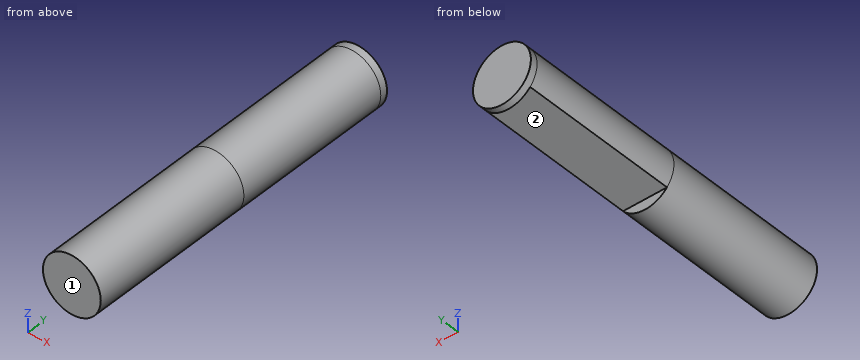
```python
from build123d import *

# Parameters (mm, degrees)
SKETCH1_R           = 8
BOSS_EXTRUDE1_DEPTH = 46
BOSS_EXTRUDE2_DEPTH = 44
SKETCH3_R           = 8
BOSS_EXTRUDE3_DEPTH = 2


with BuildPart() as part:
    # Sketch1 → Boss-Extrude1 (new body)
    with BuildSketch(Plane(origin=(0, 0, 0), x_dir=(1, 0, 0), z_dir=(0, 1, 0))):
        Circle(SKETCH1_R)
    extrude(amount=BOSS_EXTRUDE1_DEPTH)

    # Sketch2 → Boss-Extrude2 (add)
    with BuildSketch(Plane(origin=(0, 46, 0), x_dir=(1, 0, 0), z_dir=(0, 1, 0))):
        with BuildLine():
            Line((-6.079473661, 5.2), (6.079473661, 5.2))
            ThreePointArc((6.079473661, 5.2), (0, -8), (-6.079473661, 5.2))
        make_face()
    extrude(amount=BOSS_EXTRUDE2_DEPTH)

    # Sketch3 → Boss-Extrude3 (add)
    with BuildSketch(Plane(origin=(0, 90, 0), x_dir=(1, 0, 0), z_dir=(0, 1, 0))):
        Circle(SKETCH3_R)
    extrude(amount=BOSS_EXTRUDE3_DEPTH)


solid = part.part
```
Model file for the job. Use its own axes, mm. Face numbers are marked on the shaded views. A direction names the side the tool comes from. Round coordinates to 2 decimals unless told otherwise and drop trailing zeros. Write each loop counter-clockwise with the first axis right and the second up, starting at its lowest first coordinate (ties: lowest second). Pieces come first, ordered by that corner, then holes. Notation, with made-up numbers: (43.5, -31.5) - (87.5, -31.5) arc R31 ccw to (87.5, 1.5) - close; hole circle Ø7 at (-15, 31.25). An arc over 180 degrees is marked (long way). Use CSV: the item, a comma, the result in double quotes. Start each with the question number.
Item 1: Drill centre lines: L1, parallel to Y at x = -3.75, z = -6; L2, parallel to Z at x = -4, y = 18; L3, parallel to X at y = 8, z = 3.5. Where is each one in solid material? Low to high. Write a range as [from, to].
Item 2: Tool access for the marked faces 1 and 2: list every direction of +Z, -Z, +X, -X, +Y, -Y with a clear straight run to the whole face (end or side of a thin tool).
Item 3: Pin check, flat tips, straight feed: P1, Ø3, axis at x = 2, z = -7, coming from the -Y side; P2, Ø1.5, axis at y = 73.5, z = 1, coming from the -X side; P3, Ø6, axis at x = -6, y = 33.5, coming from the +Z side; P4, Ø1.5, axis at y = 59.5, z = -2.5, coming from the -X side. Stop position of each tip, or through.
Item 4: Band-saw the part on B-B (y = 8.5). Write the cut outline in (x, z).
Item 5: Band-saw the part on A-A (x = 0). Write the cut outline in (y, z).
Item 6: Band-saw the part on D-D (z = 1.75). Write the cut outline in (x, y), and give its area (3 significant figures).
Item 7: Band-saw the part on C-C (z = 6). Write the cut outline in (x, y).
Checked values:
1,L1,"y = [0, 46], [90, 92]"
1,L2,"z = [-6.93, 6.93]"
1,L3,"x = [-7.19, 7.19]"
2,face 1,"+Z, -Z, +X, -X, -Y"
2,face 2,"-Z, +X, -X"
3,P1,"stops at y = 0"
3,P2,"stops at x = -8"
3,P3,"stops at z = 7.42"
3,P4,"stops at x = -7.81"
4,outline,"circle Ø16 at (0, 0)"
5,outline,"(0, -8) - (46, -8) - (46, -5.2) - (90, -5.2) - (90, -8) - (92, -8) - (92, 8) - (0, 8) - close"
6,outline,"(-7.81, 0) - (7.81, 0) - (7.81, 92) - (-7.81, 92) - close"
6,area,"1,440 mm²"
7,outline,"(-5.29, 0) - (5.29, 0) - (5.29, 92) - (-5.29, 92) - close"
